Source: three-view drawing plus pictorial views. Frame: mm from the lowest corner of the part. Round coordinates to 2 decimals unless told otherwise and drop trailing zeros. Write each loop counter-clockwise with the first axis right and the second up, starting at its lowest first coordinate (ties: lowest second). Pieces come first, ordered by that corner, then holes. Notation, with made-up numbers: M 67.25,75.5 L 77.25,75.5 A11 cw 77.25,88.5 Z; hole C 15,42 d3. An arc over 180 degrees is marked long. Answer as CSV lines item,"result". Start each with the question number.
Q1. Ray query, probe 1 along Y at (x, z) = (10.25, 7); probe 2 along Z at (x, y) = (10.25, 47); probe 3 along X at (y, z) = (59, 6.5). Return the intervals inside material, ascending.
Q2. Mould query, pull axis Y, two halves, no side actions, for the marked faces 1, 2, 3 and 4. Classes: pulls with the +Y half, pulls with the -Y half, needs draft (parallel to the pull), parting line crosses it, or undercut.
Q3. Section query C-C on y = 80. Output: boundary loops of the cut face in (x, z), and give its area (3 significant figures).
Q4. First-contact query: pin 1 (4 mm diameter, centred on x = 22, y = 26, fed in from +Z). Flat tip, straight axial feed; report the tip coordinate or a pass-through.
Q5. Section query B-B on y = 38.1. Output: boundary loops of the cut face in (x, z), and give its area (3 significant figures).
Q6. Section query A-A on x = 12.7. Output: boundary loops of the cut face in (y, z).
Q7. Section query D-D on x = 3. Output: boundary loops of the cut face in (y, z), and give its area (3 significant figures).
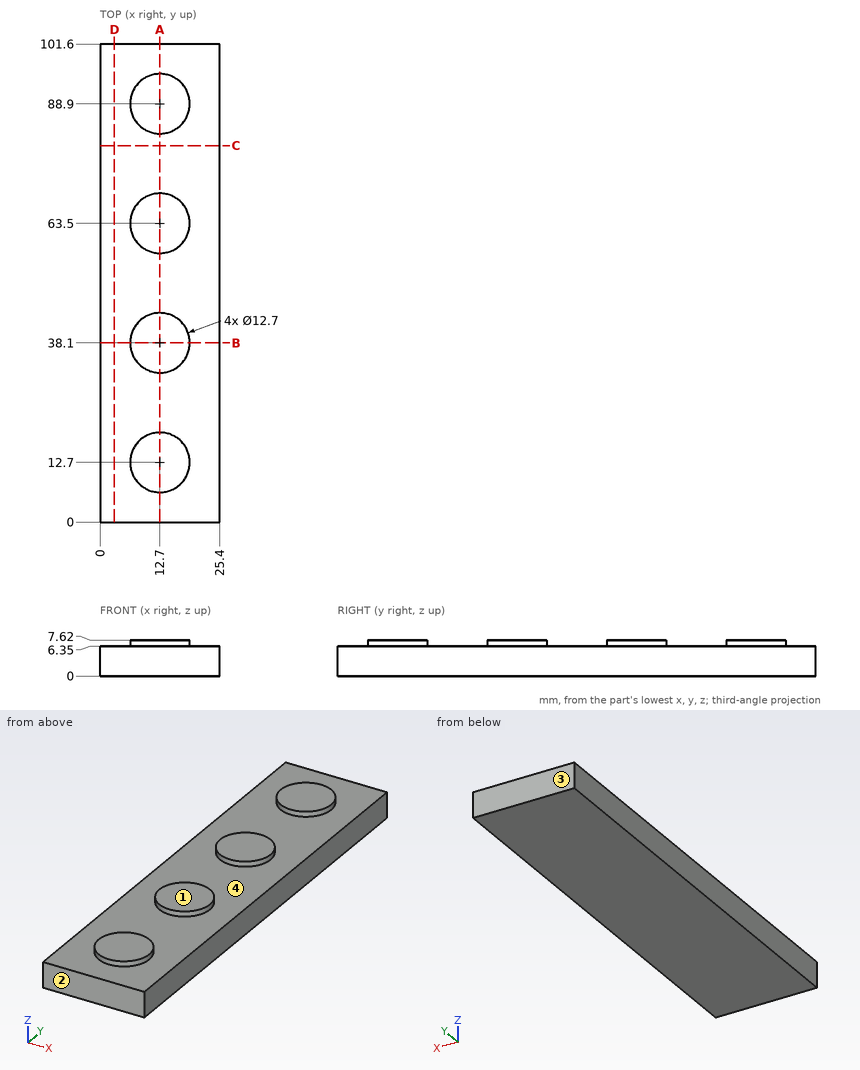
Entries:
1,probe 1,"y = 6.84 to 18.56, 32.24 to 43.96, 57.64 to 69.36, 83.04 to 94.76"
1,probe 2,"z = 0 to 6.35"
1,probe 3,"x = 8.22 to 17.18"
2,face 1,"needs draft"
2,face 2,"pulls with the -Y half"
2,face 3,"pulls with the +Y half"
2,face 4,"undercut"
3,outline,"M 0,0 L 25.4,0 L 25.4,6.35 L 0,6.35 Z"
3,area,"161 mm^2"
4,pin 1,"stops at z = 6.35"
5,outline,"M 0,0 L 25.4,0 L 25.4,6.35 L 19.05,6.35 L 19.05,7.62 L 6.35,7.62 L 6.35,6.35 L 0,6.35 Z"
5,area,"177 mm^2"
6,outline,"M 0,0 L 101.6,0 L 101.6,6.35 L 95.25,6.35 L 95.25,7.62 L 82.55,7.62 L 82.55,6.35 L 69.85,6.35 L 69.85,7.62 L 57.15,7.62 L 57.15,6.35 L 44.45,6.35 L 44.45,7.62 L 31.75,7.62 L 31.75,6.35 L 19.05,6.35 L 19.05,7.62 L 6.35,7.62 L 6.35,6.35 L 0,6.35 Z"
7,outline,"M 0,0 L 101.6,0 L 101.6,6.35 L 0,6.35 Z"
7,area,"645 mm^2"
